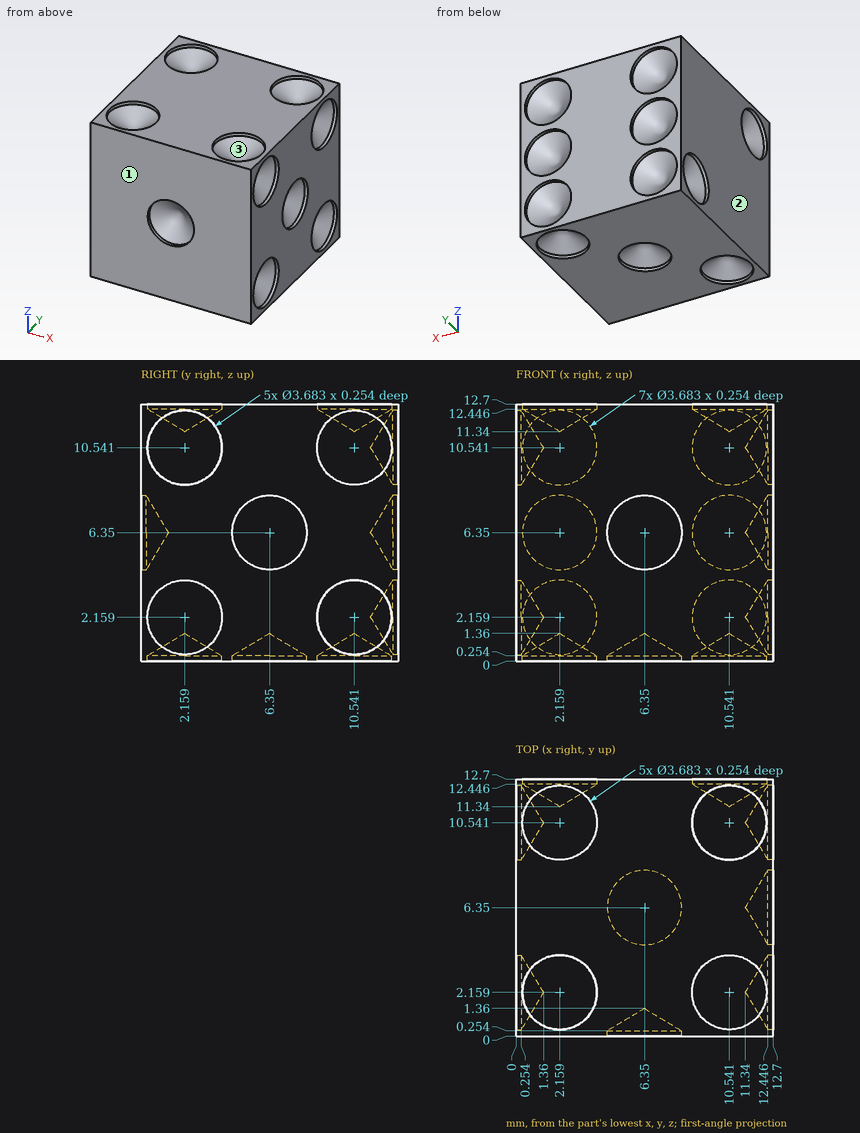
Print and shaded views of the part. All mm, measured from the part's lowest x, y and z. Give positions to 0.01 mm unless a question says otherwise; leave off trailing zeros. Answer in a Markdown table with one row per item.
Item 1: Probe line 1 along X through (y, z) = (12.5, 6.35); line 2 along X through (y, z) = (0.1, 6.35). List the from-to ranges inside material, lowest first. Write a range as [from, to].
Findings below:
| item | result |
|---|---|
| line 1 | x = [0, 0.32], [4, 8.7], [12.38, 12.7] |
| line 2 | x = [0, 4.51], [8.19, 12.7] |
Item 2: Flat gauge pins, fed straight in: P1, Ø5, axis at x = 10.541, z = 10.541, coming from the -Y side; P2, Ø3.5, axis at x = 2.159, z = 2.159, coming from the +Y side; P3, Ø3.5, axis at y = 2.159, z = 2.159, coming from the +X side; P4, Ø2, axis at y = 10.541, z = 2.159, coming from the +X side. Where does each tip first touch, or does it go through?
Findings below:
| item | result |
|---|---|
| P1 | stops at y = 0 |
| P2 | stops at y = 12.39 |
| P3 | stops at x = 12.39 |
| P4 | stops at x = 11.94 |
Item 3: Mould opens along X. For the marked faces 1, 2 and 3 say: pulls with the +X half, pulls with the -X half, needs draft (parallel to the pull), parting line crosses it, or undercut.
Findings below:
| item | result |
|---|---|
| face 1 | needs draft |
| face 2 | pulls with the -X half |
| face 3 | undercut |
